```python
from build123d import *

# Parameters (mm, degrees)
F2_W     = 6.35
F2_H     = 6.35
F3_DEPTH = 6.35
F5_DEPTH = 12.7
F6_R     = 5.08
F7_SIZE  = 0.508


with BuildPart() as f1:
    # F0 (on Top) → F1 (revolve)
    with BuildSketch(Plane.XY):
        Polygon((0, 6.35), (0, 0), (25.4, 0), (25.4, 8.89), (12.7, 8.89), (6.35, 6.35), align=None)
    revolve(axis=Axis((-3.302, 0, 0), (-1, 0, 0)))

    # F2 (on face) → F3 (cut)
    with BuildSketch(Plane(origin=(0, 0, 0), x_dir=(0, -1, 0), z_dir=(-1, 0, 0))):
        Rectangle(F2_W, F2_H)
    extrude(amount=-F3_DEPTH, mode=Mode.SUBTRACT)

    # F4 (on face) → F5 (cut)
    with BuildSketch(Plane.YZ.offset(25.4)):
        Polygon((7.332348, 0), (3.666174, 6.35), (-3.666174, 6.35), (-7.332348, 0), (-3.666174, -6.35), (3.666174, -6.35), align=None)
    extrude(amount=-F5_DEPTH, mode=Mode.SUBTRACT)

    # F6
    f6_edges = [f1.edges().sort_by_distance(p)[0] for p in [
        (12.7, -8.89, 0),
        (6.35, -6.35, 0),
    ]]
    fillet(f6_edges, radius=F6_R)

    # F7
    f7_edges = [f1.edges().sort_by_distance(p)[0] for p in [
        (25.4, -8.89, 0),
        (0, -6.35, 0),
    ]]
    chamfer(f7_edges, length=F7_SIZE)


solid = f1.part
```
CAD build for the part. Positions are in the model's coordinates, mm. A direction names the side the tool comes from. Round coordinates to 2 decimals unless told otherwise and drop trailing zeros. Loops run counter-clockwise (first coordinate to the right, second up) from the corner with the lowest first, then second, coordinate; pieces in that order, holes last. Notation, with made-up numbers: M -26.5,-5 L 32.5,-5 A34 cw 32.5,28 Z; hole C 3,64.5 d10. An arc over 180 degrees is marked long. Return JSON: item names as keys, results as strings. Group by question number.
(1) Saw through at A-A, the plane x = 16.75. List the corners of the cut face in (y, z), and give its area (3 significant figures).
(2) Tool access for faces 4 (the flat face through (25.4, 6, -3)), 5 (the flat face through (19.139, 5.525, 3.131)), 6 (the flat face through (6.35, 0, 0)): list every direction of +Z, -Z, +X, -X, +Y, -Y with a clear straight run to the whole face (end or side of a thin tool).
(3) Mould opens along Z. For faces 1 (the flat face through (19, 0, -6.35)), 2 (the cylindrical face through (19.21, -1.93, 8.68)), 3 (the flat face through (0, 0, 4)) say: +Z half, -Z half, draft (parallel to the pull), parting line (faces both ways), or undercut.
(4) Drop flat-ended pins along their axis: P1, Ø7, axis at x = 3.5, y = -1, coming from the +Z side; P2, Ø2, axis at x = 19.5, y = 4, coming from the +Z side; P3, Ø5, axis at x = 13.5, y = 5, coming from the +Z side. Give the stop position or say it passes through.
(5) Wall check: probe 1 along Y at (x, z) = (4.25, -2.5) (3 decimals); probe 2 along Z at (x, y) = (21, 2.5); probe 3 along Z at (x, y) = (21.5, 0). Give the ranges that are in metal, low to high. Write a range as [from, to].
Answer list:
{
 "1": {"outline": "C 0,0 d17.78; hole M -7.33,0 L -3.67,-6.35 L 3.67,-6.35 L 7.33,0 L 3.67,6.35 L -3.67,6.35 Z", "area": "109 mm2"},
 "2": {"face 4": "+Z, -Z, +X, +Y, -Y", "face 5": "+X", "face 6": "-X"},
 "3": {"face 1": "undercut", "face 2": "parting line", "face 3": "draft"},
 "4": {"P1": "z = 6.59", "P2": "z = 8.37", "P3": "z = 8.53"},
 "5": {"probe 1": "[-5.837, -3.175], [3.175, 5.837]", "probe 2": "[-8.53, -6.35], [6.35, 8.53]", "probe 3": "[-8.89, -6.35], [6.35, 8.89]"}
}
